from build123d import *

# Parameters (mm, degrees)
SKETCH1_R               = 12.7
BOSS_EXTRUDE2_DEPTH     = 3.302
SKETCH4_R               = 0.744786443
CUT_EXTRUDE4_DEPTH      = 140.7
CUT_EXTRUDE4_DEPTH_BACK = 140.7


with BuildPart() as part:
    # Sketch1 → Boss-Extrude2 (new body)
    with BuildSketch(Plane(origin=(0, 0, 0), x_dir=(1, 0, 0), z_dir=(0, 1, 0))):
        with BuildLine():
            ThreePointArc((139.7, 0), (-12.753253462, 139.116657975), (-137.371503595, -25.4))
            Line((-137.371503595, -25.4), (137.371503595, -25.4))
            ThreePointArc((137.371503595, -25.4), (139.116657975, -12.753253462), (139.7, 0))
        make_face()
        Circle(SKETCH1_R, mode=Mode.SUBTRACT)
    extrude(amount=BOSS_EXTRUDE2_DEPTH)

    # Sketch4 → Cut-Extrude4 (cut, two sides)
    with BuildSketch(Plane(origin=(0, 0, 0), x_dir=(0, 0, -1), z_dir=(1, 0, 0))) as cut_extrude4_sk:
        with Locations((-23.622, 1.524)):
            Circle(SKETCH4_R)
    extrude(amount=CUT_EXTRUDE4_DEPTH, mode=Mode.SUBTRACT)
    extrude(cut_extrude4_sk.sketch, amount=-CUT_EXTRUDE4_DEPTH_BACK, mode=Mode.SUBTRACT)


solid = part.part
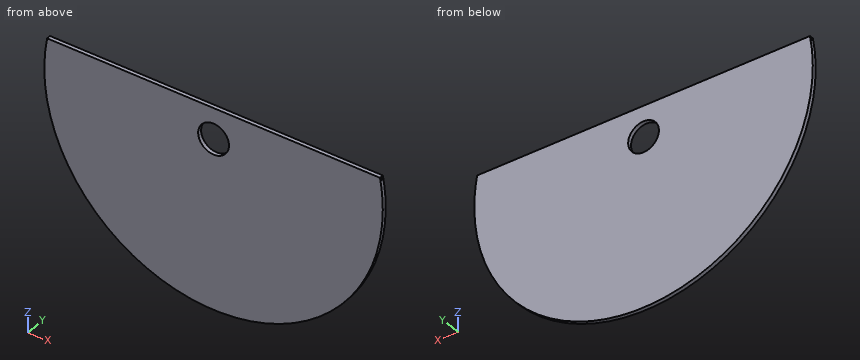
Can you work these out from the model? Positions are in its coordinate system, mm. Give positions to 0.01 mm unless a question says otherwise; leave off trailing zeros. Order: outer loops, then holes, each group sorted by start corner. A loop starts at its lowest first (then second) coordinate and runs counter-clockwise, first axis right, second up. Notation, with made-up numbers: M -24,-1.75 L -4,-1.75 A25 ccw -4,19.25 Z; hole C 31,-24.5 d10. An arc over 180 degrees is marked long. Use one line per item in the form item = value.
Item 1: If I drill on line 1 along Z through (x, y) = (0, 1.65); line 2 along X through (y, z) = (1.05, 0); line 3 along Z through (x, y) = (0, 0.7), over which ranges is the centre line in solid material (lowest first)? Write a range as [from, to].
Values follow:
line_1 = [-139.7, -12.7], [12.7, 22.89], [24.36, 25.4]
line_2 = [-139.7, -12.7], [12.7, 139.7]
line_3 = [-139.7, -12.7], [12.7, 25.4]
Item 2: If we section it at A-A, the plane x = 0: Write out the boundary of the cut face in (y, z), and give its area (3 significant figures).
Values follow:
outline = M 0,-139.7 L 3.3,-139.7 L 3.3,-12.7 L 0,-12.7 Z; M 0,12.7 L 3.3,12.7 L 3.3,25.4 L 0,25.4 Z; hole C 1.52,23.62 d1.49
area = 460 mm^2
Item 3: If we section it at D-D, the plane x = -83: Write out the boundary of the cut face in (y, z), and give its area (3 significant figures).
Values follow:
outline = M 0,-112.37 L 3.3,-112.37 L 3.3,25.4 L 0,25.4 Z; hole C 1.52,23.62 d1.49
area = 453 mm^2
Item 4: If we section it at C-C, the plane z = -78.5: Write out the boundary of the cut face in (x, y), and give its area (3 significant figures).
Values follow:
outline = M -115.56,0 L 115.56,0 L 115.56,3.3 L -115.56,3.3 Z
area = 763 mm^2
Item 5: If we section it at B-B, the plane x = 73: Write out the boundary of the cut face in (y, z).
Values follow:
outline = M 0,-119.11 L 3.3,-119.11 L 3.3,25.4 L 0,25.4 Z; hole C 1.52,23.62 d1.49
